For this review, take the finished solid that the model builds, in its own axes (mm). Round coordinates to 2 decimals unless told otherwise and drop trailing zeros. Write each loop counter-clockwise with the first axis right and the second up, starting at its lowest first coordinate (ties: lowest second). Pieces come first, ordered by that corner, then holes. Notation, with made-up numbers: M -18,11.25 L 7,11.25 A31 ccw 7,39.25 Z; hole C 58,36.5 d9. An arc over 180 degrees is marked long. Use one line per item in the form item = value. Start each with the question number.
Item 1: Add section C-C (y = 49.95). State the section outline as (x, z) points, and give its area (3 significant figures).
Item 2: For P1, Ø1, axis at x = -41, y = 50, coming from the -Z side; P2, Ø1.5, axis at y = 48.5, z = -38, coming from the -X side, all flat-tipped, find the tip position at first contact; note any pin that passes through.
Item 3: Draft analysis for pull direction X (two halves, no side actions). For faces 1 (the cylindrical face through (2.64, 50.54, -59.94)), 2 (the cylindrical face through (19.52, 50.54, 62)), 3 (the flat face through (19, 48, -57.5)), state which applies: released by +X, released by -X, zero draft, split by the parting line, or undercut.
Item 4: For line 1 (X direction, y = 49.1, z = 0); line 2 (X direction, y = 48.3, z = -23); line 3 (Z direction, x = -47, y = 50.1), list the stretches that pass through material, from the lowest coordinate up. Write a range as [from, to].
Item 5: Add section A-A (z = 0). State the section outline as (x, y) points, and give its area (3 significant figures).
Item 6: Add section B-B (x = 0). State the section outline as (y, z) points.
from build123d import *

# Parameters (mm, degrees)
SKETCH1_R           = 75
SKETCH1_R_2         = 62.3
BOSS_EXTRUDE1_DEPTH = 53
BOSS_EXTRUDE3_START = 3
SKETCH3_R           = 75
SKETCH3_R_2         = 47
BOSS_EXTRUDE3_DEPTH = 3
BOSS_EXTRUDE4_START = 14
SKETCH4_R           = 50.1
SKETCH4_R_2         = 47
BOSS_EXTRUDE4_DEPTH = 14
BOSS_EXTRUDE5_START = 1
SKETCH5_R           = 62.3
SKETCH5_R_2         = 50.1
BOSS_EXTRUDE5_DEPTH = 1
CUT_EXTRUDE2_START  = -64
SKETCH6_R           = 75
SKETCH6_R_2         = 67.5
CUT_EXTRUDE2_DEPTH  = 64
BOSS_EXTRUDE6_REACH = 111.186
SKETCH7_R           = 62.3
SKETCH7_R_2         = 60
SKETCH9_R           = 50.1
SKETCH9_R_2         = 47
CUT_EXTRUDE3_DEPTH  = 17
BOSS_EXTRUDE7_START = -4
SKETCH10_R          = 50.1
SKETCH10_R_2        = 48.5
BOSS_EXTRUDE7_DEPTH = 4
SKETCH12_R          = 48.5
SKETCH12_R_2        = 47.6
BOSS_EXTRUDE8_DEPTH = 4
BOSS_EXTRUDE9_START = -17
SKETCH13_R          = 47.6
SKETCH13_R_2        = 45.1
BOSS_EXTRUDE9_DEPTH = 17
SKETCH14_R          = 75.997463879
CUT_EXTRUDE4_DEPTH  = 48
SKETCH15_R          = 79.637366743
SKETCH15_R_2        = 65
CUT_EXTRUDE5_DEPTH  = 50


with BuildPart() as part:
    # Sketch1 → Boss-Extrude1 (new body)
    with BuildSketch(Plane(origin=(0, 0, 0), x_dir=(1, 0, 0), z_dir=(0, 1, 0))):
        with Locations(Location((0, 0, 0), (0, 0, 270))):
            Circle(SKETCH1_R)
        with Locations(Location((0, 0, 0), (0, 0, 270))):
            Circle(SKETCH1_R_2, mode=Mode.SUBTRACT)
    extrude(amount=BOSS_EXTRUDE1_DEPTH)

    # Sketch3 → Boss-Extrude3 (add)
    with BuildSketch(Plane(origin=(0, 20, 0), x_dir=(-1, 0, 0), z_dir=(0, -1, 0)).offset(BOSS_EXTRUDE3_START)):
        with Locations(Location((0, 0, 0), (0, 0, 270))):
            Circle(SKETCH3_R)
        with Locations(Location((0, 0, 0), (0, 0, 90))):
            Circle(SKETCH3_R_2, mode=Mode.SUBTRACT)
    extrude(amount=-BOSS_EXTRUDE3_DEPTH)

    # Sketch4 → Boss-Extrude4 (add)
    with BuildSketch(Plane.XZ.offset(-17).offset(BOSS_EXTRUDE4_START)):
        with Locations(Location((0, 0, 0), (0, 0, 270))):
            Circle(SKETCH4_R)
        with Locations(Location((0, 0, 0), (0, 0, 270))):
            Circle(SKETCH4_R_2, mode=Mode.SUBTRACT)
    extrude(amount=-BOSS_EXTRUDE4_DEPTH)

    # Sketch5 → Boss-Extrude5 (add)
    with BuildSketch(Plane.XZ.offset(-17).offset(BOSS_EXTRUDE5_START)):
        with Locations(Location((0, 0, 0), (0, 0, 270))):
            Circle(SKETCH5_R)
        with Locations(Location((0, 0, 0), (0, 0, 270))):
            Circle(SKETCH5_R_2, mode=Mode.SUBTRACT)
    extrude(amount=-BOSS_EXTRUDE5_DEPTH)

    # Sketch6 → Cut-Extrude2 (cut)
    with BuildSketch(Plane(origin=(0, 53, 0), x_dir=(1, 0, 0), z_dir=(0, 1, 0)).offset(CUT_EXTRUDE2_START)):
        Circle(SKETCH6_R)
        with Locations(Location((0, 0, 0), (0, 0, 270))):
            Circle(SKETCH6_R_2, mode=Mode.SUBTRACT)
    extrude(amount=CUT_EXTRUDE2_DEPTH, mode=Mode.SUBTRACT)

    # Boss-Extrude6: up to this face of the body (flat: up to its plane)
    boss_extrude6_end = Plane(part.part.faces().sort_by_distance((0, 0, -65.590811691))[0])
    # Sketch7 → Boss-Extrude6 (add, up to the picked face)
    with BuildSketch(Plane(origin=(0, 53, 0), x_dir=(1, 0, 0), z_dir=(0, 1, 0)), mode=Mode.PRIVATE) as boss_extrude6_sk1:
        Circle(SKETCH7_R)
        with Locations(Location((0, 0, 0), (0, 0, 270))):
            Circle(SKETCH7_R_2, mode=Mode.SUBTRACT)
    boss_extrude6_tool1 = split(extrude(boss_extrude6_sk1.sketch, amount=-BOSS_EXTRUDE6_REACH, mode=Mode.PRIVATE), bisect_by=boss_extrude6_end, keep=Keep.BOTH, mode=Mode.PRIVATE)
    add(boss_extrude6_tool1.solids().sort_by(Axis((-60.53789, 53, 0), (0, -1, 0)))[0])

    # Sketch9 → Cut-Extrude3 (cut)
    with BuildSketch(Plane.XZ.offset(-3)):
        with Locations(Location((0, 0, 0), (0, 0, 270))):
            Circle(SKETCH9_R)
        Circle(SKETCH9_R_2, mode=Mode.SUBTRACT)
    extrude(amount=-CUT_EXTRUDE3_DEPTH, mode=Mode.SUBTRACT)

    # Sketch10 → Boss-Extrude7 (add)
    with BuildSketch(Plane(origin=(0, 20, 0), x_dir=(1, 0, 0), z_dir=(0, 1, 0)).offset(BOSS_EXTRUDE7_START)):
        Circle(SKETCH10_R)
        with Locations(Location((0, 0, 0), (0, 0, 270))):
            Circle(SKETCH10_R_2, mode=Mode.SUBTRACT)
    extrude(amount=BOSS_EXTRUDE7_DEPTH)

    # Sketch12 → Boss-Extrude8 (add)
    with BuildSketch(Plane.XZ.offset(-16)):
        Circle(SKETCH12_R)
        with Locations(Location((0, 0, 0), (0, 0, 270))):
            Circle(SKETCH12_R_2, mode=Mode.SUBTRACT)
    extrude(amount=-BOSS_EXTRUDE8_DEPTH)

    # Sketch13 → Boss-Extrude9 (add)
    with BuildSketch(Plane(origin=(0, 20, 0), x_dir=(1, 0, 0), z_dir=(0, 1, 0)).offset(BOSS_EXTRUDE9_START)):
        with Locations(Location((0, 0, 0), (0, 0, 270))):
            Circle(SKETCH13_R)
        with Locations(Location((0, 0, 0), (0, 0, 270))):
            Circle(SKETCH13_R_2, mode=Mode.SUBTRACT)
    extrude(amount=BOSS_EXTRUDE9_DEPTH)

    # Sketch14 → Cut-Extrude4 (cut)
    with BuildSketch(Plane.XZ):
        Circle(SKETCH14_R)
    extrude(amount=-CUT_EXTRUDE4_DEPTH, mode=Mode.SUBTRACT)

    # Sketch15 → Cut-Extrude5 (cut)
    with BuildSketch(Plane(origin=(0, 53, 0), x_dir=(1, 0, 0), z_dir=(0, 1, 0))):
        Circle(SKETCH15_R)
        with Locations(Location((0, 0, 0), (0, 0, 270))):
            Circle(SKETCH15_R_2, mode=Mode.SUBTRACT)
    extrude(amount=-CUT_EXTRUDE5_DEPTH, mode=Mode.SUBTRACT)


solid = part.part
Calculated:
q1.outline = C 0,0 d130; hole C 0,0 d120
q1.area = 1,960 mm^2
q2.P1 = -50.84
q2.P2 = -53.27
q3.face_1 = undercut
q3.face_2 = split by the parting line
q3.face_3 = zero draft
q4.line_1 = [-65, -60], [60, 65]
q4.line_2 = [-60.79, -55.42], [55.42, 60.79]
q4.line_3 = [-44.9, -37.3], [37.3, 44.9]
q5.outline = M -65,48 L -60,48 L -60,53 L -65,53 Z; M 60,48 L 65,48 L 65,53 L 60,53 Z
q5.area = 50.0 mm^2
q6.outline = M 48,-65 L 53,-65 L 53,-60 L 48,-60 Z; M 48,60 L 53,60 L 53,65 L 48,65 Z
